Check sheet for the modelled part. Datum: model origin and axes. Units: mm. A direction names the side the tool comes from. Coordinates: 2 decimals unless noted, no trailing zeros. Loops run counter-clockwise (first coordinate to the right, second up) from the corner with the lowest first, then second, coordinate; pieces in that order, holes last.
from build123d import *

# Parameters (mm, degrees)
SKETCH1_W           = 109.2835
SKETCH1_H           = 61.8236
SKETCH1_R           = 1.27
SKETCH1_R_2         = 1.5875
BOSS_EXTRUDE1_DEPTH = 3.175
BOSS_EXTRUDE2_START = -40.005
SKETCH3_R           = 1.5875
BOSS_EXTRUDE2_DEPTH = 40.005
SKETCH4_W           = 90.288549843
SKETCH4_H           = 56.7436
CUT_EXTRUDE1_DEPTH  = 1.905
FILLET1_R           = 2.54
SKETCH6_R           = 1.27
BOSS_EXTRUDE3_DEPTH = 5.08
FILLET2_R           = 2.54
SKETCH9_R           = 1.778
CUT_EXTRUDE4_DEPTH  = 3.81
CUT_EXTRUDE5_DEPTH  = 3.556


with BuildPart() as part:
    # Sketch1 → Boss-Extrude1 (new body)
    with BuildSketch(Plane.XY):
        Rectangle(SKETCH1_W, SKETCH1_H)
        with Locations((30.51175, 23.9268)):
            Circle(SKETCH1_R, mode=Mode.SUBTRACT)
        with Locations((-20.28825, 8.6868)):
            Circle(SKETCH1_R, mode=Mode.SUBTRACT)
        with Locations((-20.28825, -19.2532)):
            Circle(SKETCH1_R, mode=Mode.SUBTRACT)
        with Locations((31.78175, -24.3332)):
            Circle(SKETCH1_R, mode=Mode.SUBTRACT)
        with Locations((50.83175, -27.1018)):
            Circle(SKETCH1_R_2, mode=Mode.SUBTRACT)
        with Locations((-49.16805, 25.4381)):
            Circle(SKETCH1_R_2, mode=Mode.SUBTRACT)
        with Locations((-49.10175, -25.8718)):
            Circle(SKETCH1_R_2, mode=Mode.SUBTRACT)
        with Locations(Location((50.83175, 27.1018, 0), (0, 0, 180))):
            Circle(SKETCH1_R_2, mode=Mode.SUBTRACT)
    extrude(amount=BOSS_EXTRUDE1_DEPTH)

    # Sketch3 → Boss-Extrude2 (add)
    # profile 1 of 3: a face of its own
    with BuildSketch(Plane.XY.offset(BOSS_EXTRUDE2_START)):
        with BuildLine():
            Line((-54.64175, 30.9118), (-41.94175, 30.9118))
            Line((-41.94175, 30.9118), (-41.94175, 28.3718))
            Line((-41.94175, 28.3718), (-47.953953912, 28.3718))
            ThreePointArc((-47.953953912, 28.3718), (-46.92298597, 23.19303597), (-52.10175, 24.224003912))
            Line((-52.10175, 24.224003912), (-52.10175, 18.2118))
            Line((-52.10175, 18.2118), (-52.10175, -18.2118))
            Line((-52.10175, -18.2118), (-52.10175, -24.832268856))
            ThreePointArc((-52.10175, -24.832268856), (-47.256776002, -23.28786967), (-47.144551747, -28.3718))
            Line((-47.144551747, -28.3718), (-41.94175, -28.3718))
            Line((-41.94175, -28.3718), (-41.94175, -30.9118))
            Line((-41.94175, -30.9118), (-54.64175, -30.9118))
            Line((-54.64175, -30.9118), (-54.64175, -18.2118))
            Line((-54.64175, -18.2118), (-54.64175, 18.2118))
            Line((-54.64175, 18.2118), (-54.64175, 30.9118))
        make_face()
        with Locations((-49.16805, 25.4381)):
            Circle(SKETCH3_R, mode=Mode.SUBTRACT)
        with Locations((-49.10175, -25.8718)):
            Circle(SKETCH3_R, mode=Mode.SUBTRACT)
    # profile 2 of 3: a face of its own
    with BuildSketch(Plane.XY.offset(BOSS_EXTRUDE2_START)):
        with BuildLine():
            Line((54.64175, 30.9118), (54.64175, 18.2118))
            Line((54.64175, 18.2118), (52.10175, 18.2118))
            Line((52.10175, 18.2118), (52.10175, 22.49507603))
            ThreePointArc((52.10175, 22.49507603), (47.452785237, 23.722835237), (46.22502603, 28.3718))
            Line((46.22502603, 28.3718), (41.94175, 28.3718))
            Line((41.94175, 28.3718), (41.94175, 30.9118))
            Line((41.94175, 30.9118), (54.64175, 30.9118))
        make_face()
        with Locations(Location((50.83175, 27.1018, 0), (0, 0, 180))):
            Circle(SKETCH3_R, mode=Mode.SUBTRACT)
    # profile 3 of 3: a face of its own
    with BuildSketch(Plane.XY.offset(BOSS_EXTRUDE2_START)):
        with BuildLine():
            Line((52.10175, -24.191864434), (52.10175, -18.2118))
            Line((52.10175, -18.2118), (54.64175, -18.2118))
            Line((54.64175, -18.2118), (54.64175, -30.9118))
            Line((54.64175, -30.9118), (41.94175, -30.9118))
            Line((41.94175, -30.9118), (41.94175, -28.3718))
            Line((41.94175, -28.3718), (47.921814434, -28.3718))
            ThreePointArc((47.921814434, -28.3718), (48.58668597, -24.85673597), (52.10175, -24.191864434))
        make_face()
        with Locations((50.83175, -27.1018)):
            Circle(SKETCH3_R, mode=Mode.SUBTRACT)
    extrude(amount=BOSS_EXTRUDE2_DEPTH)

    # Sketch4 → Cut-Extrude1 (cut)
    with BuildSketch(Plane(origin=(0, 0, -40.005), x_dir=(-1, 0, 0), z_dir=(0, 0, -1))):
        with Locations((6.957475078, 0)):
            Rectangle(SKETCH4_W, SKETCH4_H)
    extrude(amount=-CUT_EXTRUDE1_DEPTH, mode=Mode.SUBTRACT)

    # Fillet1
    fillet1_edges = [part.edges().sort_by_distance(p)[0] for p in [
        (52.10175, 22.49507603, -20.0025),
        (46.22502603, 28.3718, -20.0025),
        (-47.144551747, -28.3718, -19.05),
        (-52.10175, -24.832268856, -19.05),
        (-52.10175, 24.224003912, -19.05),
        (-47.953953912, 28.3718, -19.05),
        (-54.64175, 30.9118, -18.415),
        (54.64175, 30.9118, -18.415),
        (54.64175, -30.9118, -18.415),
        (-54.64175, -30.9118, -18.415),
        (47.921814434, -28.3718, -20.0025),
        (52.10175, -24.191864434, -20.0025),
    ]]
    fillet(fillet1_edges, radius=FILLET1_R)

    # Sketch6 → Boss-Extrude3 (add)
    with BuildSketch(Plane.XY):
        with Locations((-40.60825, 15.6718)):
            Circle(SKETCH6_R)
        with Locations((-40.60825, -15.6718)):
            Circle(SKETCH6_R)
    extrude(amount=-BOSS_EXTRUDE3_DEPTH)

    # Fillet2
    fillet2_edges = [part.edges().sort_by_distance(p)[0] for p in [
        (41.94175, 29.6418, 0),
        (53.37175, 18.2118, 0),
        (-41.94175, -29.6418, 0),
        (-41.94175, 29.6418, 0),
        (53.37175, -18.2118, 0),
        (41.94175, -29.6418, 0),
    ]]
    fillet(fillet2_edges, radius=FILLET2_R)

    # Sketch9 → Cut-Extrude4 (cut)
    with BuildSketch(Plane.ZY.offset(54.64175)):
        with Locations((-30.58287, 9.525)):
            Circle(SKETCH9_R)
        with Locations((-30.58287, -9.525)):
            Circle(SKETCH9_R)
        with BuildLine():
            Line((-12.96162, 2.54), (-12.96162, -2.54))
            ThreePointArc((-12.96162, -2.54), (-14.86662, -4.445), (-16.77162, -2.54))
            Line((-16.77162, -2.54), (-16.77162, 2.54))
            ThreePointArc((-16.77162, 2.54), (-14.86662, 4.445), (-12.96162, 2.54))
        make_face()
    extrude(amount=-CUT_EXTRUDE4_DEPTH, mode=Mode.SUBTRACT)

    # Sketch10 → Cut-Extrude5 (cut)
    with BuildSketch(Plane.XY.offset(3.175)):
        Polygon((-49.16805, 28.297715883), (-51.64455, 26.867907942), (-51.64455, 24.008292058), (-49.16805, 22.578484117), (-46.69155, 24.008292058), (-46.69155, 26.867907942), align=None)
        Polygon((-46.62525, -24.441992058), (-49.10175, -23.012184117), (-51.57825, -24.441992058), (-51.57825, -27.301607942), (-49.10175, -28.731415883), (-46.62525, -27.301607942), align=None)
        Polygon((47.972134117, 27.1018), (49.401942058, 24.6253), (52.261557942, 24.6253), (53.691365883, 27.1018), (52.261557942, 29.5783), (49.401942058, 29.5783), align=None)
        Polygon((49.401942058, -24.6253), (47.972134117, -27.1018), (49.401942058, -29.5783), (52.261557942, -29.5783), (53.691365883, -27.1018), (52.261557942, -24.6253), align=None)
    extrude(amount=-CUT_EXTRUDE5_DEPTH, mode=Mode.SUBTRACT)


solid = part.part
(1) Section check B-B, the plane x = -9.5. Enter the section's corners in (y, z) (3 decimals), plus the area to 3 significant figures.
(2) Scan lines: line 1 along X through (y, z) = (-19.5, -3.5); line 2 along X through (y, z) = (-25, -20); line 3 along Y through (x, z) = (-43.5, -27). Record each from-to range of solid material in increasing order.
(3) Draft check along Z on faces 5 (the face through (51, 29, -0.381)), 6 (the face through (-53.39, -4.445, -14.825)), 7 (the face through (53.39, -17.448, -0.724)), 8 (the face through (51.52, 21.51, -19.72)). Enter one of: pulls with the +Z half, pulls with the -Z half, needs draft (parallel to the pull), parting line crosses it, or undercut.
(4) Section check A-A, the plane z = -20. Count the separate pieces of the cut face and the enclosed holes in it, plus the area to 3 significant figures.
(5) Section check C-C, the plane y = -13. Enter the section's corners in (x, z) (3 decimals), plus the area to 3 significant figures.
(6) Set-up check for faces 1 (the face through (-51.645, 25, 1)), 2 (the face through (-41.217, 29.624, -0.764)), 3 (the face through (-46.896, 23.22, -19.317)), 4 (the face through (-19.115, 8.2, 1.565)): record each of +Z, -Z, +X, -X, +Y, -Y from which the full face is reachable in a straight line by a thin tool's end or side.
(7) Gauge pin test, flat ends, axial feed: P1, Ø3.5, axis at x = -20.29, y = 8.69, coming from the +Z side (3 decimals); P2, Ø5.5, axis at y = -9.52, z = -30.58, coming from the +X side; P3, Ø1.9, axis at x = 50.83, y = 27.1, coming from the +Z side; P4, Ø10, axis at x = -0.5, y = 15.5, coming from the -Z side. Record the tip position at first contact, or that the pin passes through.
Determined:
1. outline: (-30.912, 0) - (30.912, 0) - (30.912, 3.175) - (-30.912, 3.175) - close
1. area: 196 mm2
2. line 1: x = -54.64 to -52.1, 52.1 to 54.64
2. line 2: x = -54.64 to -50.43, -47.78 to -46.05, 48.45 to 54.64
2. line 3: y = -30.91 to -28.37, 28.37 to 30.91
3. face 5: pulls with the +Z half
3. face 6: undercut
3. face 7: pulls with the -Z half
3. face 8: needs draft
4. separate pieces: 3
4. enclosed holes: 4
4. area: 415 mm2
5. outline: (-54.642, -40.005) - (-52.102, -40.005) - (-52.102, 0) - (54.642, 0) - (54.642, 3.175) - (-54.642, 3.175) - close
5. area: 449 mm2
6. face 1: +Z
6. face 2: -Z, +Y
6. face 3: -Z
6. face 4: +Z, -Z
7. P1: stops at z = 3.175
7. P2: stops at x = -52.1
7. P3: passes through
7. P4: stops at z = 0
